Part model, mm, in its own coordinate system. Give positions to 0.01 mm unless a question says otherwise; leave off trailing zeros. Loops run counter-clockwise (first coordinate to the right, second up) from the corner with the lowest first, then second, coordinate; pieces in that order, holes last. Notation, with made-up numbers: M -36,86 L 0,86 A28 ccw 0,107 Z; hole C 20.5,25 d4. An arc over 180 degrees is marked long. Answer in a Markdown table with one row per item.
from build123d import *

# Parameters (mm, degrees)
BOSS_EXTRUDE1_DEPTH         = 203.2
F_1_4_20_TAPPED_HOLE1_D     = 5.1054
F_1_4_20_TAPPED_HOLE1_DEPTH = 19.05
F_1_4_20_TAPPED_HOLE1_TIP   = 1.533816902


with BuildPart() as part:
    # Sketch1 → Boss-Extrude1 (new, symmetric)
    with BuildSketch(Plane(origin=(0, 0, 0), x_dir=(0, 0, -1), z_dir=(1, 0, 0))):
        Polygon((5.499261314, 0), (2.749630657, 4.7625), (-2.749630657, 4.7625), (-5.499261314, 0), (-2.749630657, -4.7625), (2.749630657, -4.7625), align=None)
    extrude(amount=BOSS_EXTRUDE1_DEPTH, both=True)

    # 1/4-20 Tapped Hole1
    with Locations(Plane.ZY.offset(203.2)):
        with Locations((0, 0)):
            Hole(F_1_4_20_TAPPED_HOLE1_D / 2, depth=F_1_4_20_TAPPED_HOLE1_DEPTH)
            with Locations((0, 0, -(F_1_4_20_TAPPED_HOLE1_DEPTH + F_1_4_20_TAPPED_HOLE1_TIP / 2))):  # 118° drill point
                Cone(0, F_1_4_20_TAPPED_HOLE1_D / 2, F_1_4_20_TAPPED_HOLE1_TIP, mode=Mode.SUBTRACT)


solid = part.part
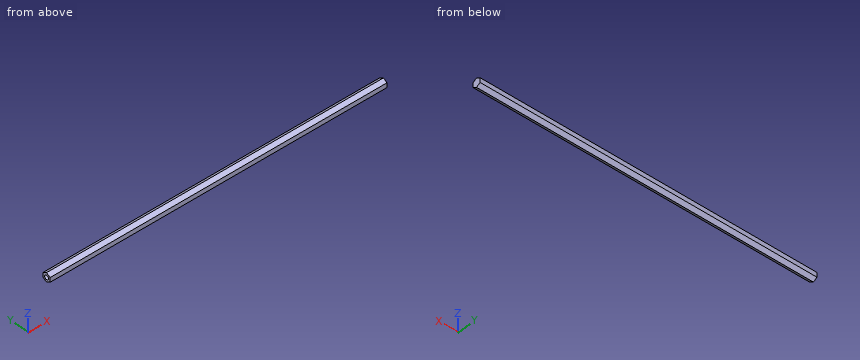
(1) Drill centre lines: line 1 along Z through (x, y) = (-198, 0); line 2 along Y through (x, z) = (-192.5, 0); line 3 along Y through (x, z) = (-143, -4). Where is each one in solid material? Low to high.
Recorded:
| item | result |
|---|---|
| line 1 | z = -5.5 to -2.55, 2.55 to 5.5 |
| line 2 | y = -4.76 to -2.55, 2.55 to 4.76 |
| line 3 | y = -2.6 to 2.6 |
(2) Saw through at A-A (x = 68). Write the cut outline in (y, z), plus the area to 3 significant figures.
Recorded:
| item | result |
|---|---|
| outline | M -4.76,-2.75 L 0,-5.5 L 4.76,-2.75 L 4.76,2.75 L 0,5.5 L -4.76,2.75 Z |
| area | 78.6 mm^2 |
(3) Pin check, flat tips, straight feed: pin 1 Ø4 at (x, y) = (-14.5, 2.5) entering from -Z; pin 2 Ø5 at (x, y) = (42.5, 1) entering from -Z; pin 3 Ø1.5 at (x, y) = (-99, 2) entering from -Z. Stop position of each tip, or through.
Recorded:
| item | result |
|---|---|
| pin 1 | stops at z = -5.21 |
| pin 2 | stops at z = -5.5 |
| pin 3 | stops at z = -4.78 |
